Here's how the part is built. I have some questions about the finished solid (model axes, mm). Round coordinates to 2 decimals unless told otherwise and drop trailing zeros. Loops run counter-clockwise (first coordinate to the right, second up) from the corner with the lowest first, then second, coordinate; pieces in that order, holes last. Notation, with made-up numbers: M 19,10 L 75,10 A13 cw 75,23 Z; hole C 29.25,42.25 d4. An arc over 180 degrees is marked long. Use a Markdown table: item, result.
from build123d import *

# Parameters (mm, degrees)
F0_R     = 3.96875
F1_DEPTH = 4.7625


with BuildPart() as f1:
    # F0 (on Front) → F1 (new body)
    with BuildSketch(Plane.XZ):
        with BuildLine():
            ThreePointArc((5.5096007047, -3.1570239268), (6.1363044447, -1.6334833218), (6.35, 0))
            ThreePointArc((6.35, 0), (6.1309371935, 1.6535141757), (5.4888632664, 3.1929422235))
            ThreePointArc((5.4888632664, 3.1929422235), (3.1570238869, 5.5096007276), (-0.0207375096, 6.3499661382))
            ThreePointArc((-0.0207375096, 6.3499661382), (-3.1929422935, 5.4888632257), (-5.5096007601, 3.1570238302))
            ThreePointArc((-5.5096007601, 3.1570238302), (-6.3499661379, -0.0207375771), (-5.4888631828, -3.1929423673))
            ThreePointArc((-5.4888631828, -3.1929423673), (-3.1570238246, -5.5096007633), (0.020737487, -6.3499661382))
            ThreePointArc((0.020737487, -6.3499661382), (3.1929422356, -5.4888632594), (5.5096007047, -3.1570239268))
        make_face()
        Circle(F0_R, mode=Mode.SUBTRACT)
        with BuildLine():
            ThreePointArc((-5.5096007601, 3.1570238302), (-3.1929422935, 5.4888632257), (-0.0207375096, 6.3499661382))
            Line((-0.0207375096, 6.3499661382), (-3.6868921494, 6.3379933427))
            Line((-3.6868921494, 6.3379933427), (-5.5096007601, 3.1570238302))
        make_face()
        with BuildLine():
            ThreePointArc((-5.4888631828, -3.1929423673), (-6.3499661379, -0.0207375771), (-5.5096007601, 3.1570238302))
            Line((-5.5096007601, 3.1570238302), (-7.3323093185, -0.023945591))
            Line((-7.3323093185, -0.023945591), (-5.4888631828, -3.1929423673))
        make_face()
        with BuildLine():
            Line((-3.6454171691, -6.3619389337), (0.020737487, -6.3499661382))
            ThreePointArc((0.020737487, -6.3499661382), (-3.1570238246, -5.5096007633), (-5.4888631828, -3.1929423673))
            Line((-5.4888631828, -3.1929423673), (-3.6454171691, -6.3619389337))
        make_face()
        with BuildLine():
            Line((3.6868921494, -6.3379933427), (5.5096007047, -3.1570239268))
            ThreePointArc((5.5096007047, -3.1570239268), (3.1929422356, -5.4888632594), (0.020737487, -6.3499661382))
            Line((0.020737487, -6.3499661382), (3.6868921494, -6.3379933427))
        make_face()
        with BuildLine():
            ThreePointArc((5.4888632664, 3.1929422235), (6.1309371935, 1.6535141757), (6.35, 0))
            ThreePointArc((6.35, 0), (6.1363044447, -1.6334833218), (5.5096007047, -3.1570239268))
            Line((5.5096007047, -3.1570239268), (7.3323093185, 0.023945591))
            Line((7.3323093185, 0.023945591), (5.4888632664, 3.1929422235))
        make_face()
        with BuildLine():
            ThreePointArc((-0.0207375096, 6.3499661382), (3.1570238869, 5.5096007276), (5.4888632664, 3.1929422235))
            Line((5.4888632664, 3.1929422235), (3.6454171691, 6.3619389337))
            Line((3.6454171691, 6.3619389337), (-0.0207375096, 6.3499661382))
        make_face()
    extrude(amount=F1_DEPTH)


solid = f1.part
1. Imagine slicing it at B-B, the plane z = 1.25. Write out the boundary of the cut face in (x, y), then the cut area to 3 significant figures.
Answer sheet:
| item | result |
|---|---|
| outline | M -6.6,-4.76 L -3.77,-4.76 L -3.77,0 L -6.6,0 Z; M 3.77,-4.76 L 6.62,-4.76 L 6.62,0 L 3.77,0 Z |
| area | 27.1 mm2 |
2. We'd pull the mould along Y, two halves only. Please class faces 1 (the face through (3, -4.762, 3)), 2 (the face through (5.515, -2.348, 3.149)), 3 (the face through (3, 0, 3)): +Y half, -Y half, draft (parallel to the pull), parting line (faces both ways), or undercut.
Answer sheet:
| item | result |
|---|---|
| face 1 | -Y half |
| face 2 | draft |
| face 3 | +Y half |
3. For pin 1 Ø1.5 at (y, z) = (-4, -3) entering from +X; pin 2 Ø1.5 at (y, z) = (-2, -4) entering from +X; pin 3 Ø1 at (y, z) = (-2.5, 1.5) entering from +X, each with a flat end and sliding along its axis, tell me the tip position at first contact or that it passes through.
Answer sheet:
| item | result |
|---|---|
| pin 1 | x = 6.03 |
| pin 2 | x = 5.46 |
| pin 3 | x = 6.76 |
4. Imagine slicing it at D-D, the plane z = -4.25. Write out the boundary of the cut face in (x, y).
Answer sheet:
| item | result |
|---|---|
| outline | M -4.87,-4.76 L 4.88,-4.76 L 4.88,0 L -4.87,0 Z |
5. Imagine slicing it at C-C, the plane x = 1.25. Write out the boundary of the cut face in (y, z), then the cut area to 3 significant figures.
Answer sheet:
| item | result |
|---|---|
| outline | M -4.76,-6.35 L 0,-6.35 L 0,-3.77 L -4.76,-3.77 Z; M -4.76,3.77 L 0,3.77 L 0,6.35 L -4.76,6.35 Z |
| area | 24.6 mm2 |
6. Imagine slicing it at A-A, the plane y = -3.35. Write out the boundary of the cut face in (x, z).
Answer sheet:
| item | result |
|---|---|
| outline | M -7.33,-0.02 L -3.65,-6.36 L 3.69,-6.34 L 7.33,0.02 L 3.65,6.36 L -3.69,6.34 Z; hole C 0,0 d7.94 |
7. I need wall thicknesses on probe 1 along Z at (x, y) = (0, -2.25); probe 2 along Z at (x, y) = (-3.25, -3.5); probe 3 along X at (y, z) = (-1.1, 1.25). Which ranges of each line are inside material? Lowest first, please. Write a range as from..to.
Answer sheet:
| item | result |
|---|---|
| probe 1 | -6.35..-3.97, 3.97..6.35 |
| probe 2 | -6.36..-2.28, 2.28..6.34 |
| probe 3 | -6.6..-3.77, 3.77..6.62 |
